Verification items for this drawing (mm, ordinates from the low corner). A direction names the side the tool comes from. Round coordinates to 2 decimals unless told otherwise and drop trailing zeros. Loops run counter-clockwise (first coordinate to the right, second up) from the corner with the lowest first, then second, coordinate; pieces in that order, holes last. Notation, with made-up numbers: (-27.75, 78.5) - (-13.75, 78.5) arc R16 cw to (-13.75, 109.5) - close; hole circle Ø3 at (48, 9). An arc over 180 degrees is marked (long way). Write item = value, one per line.
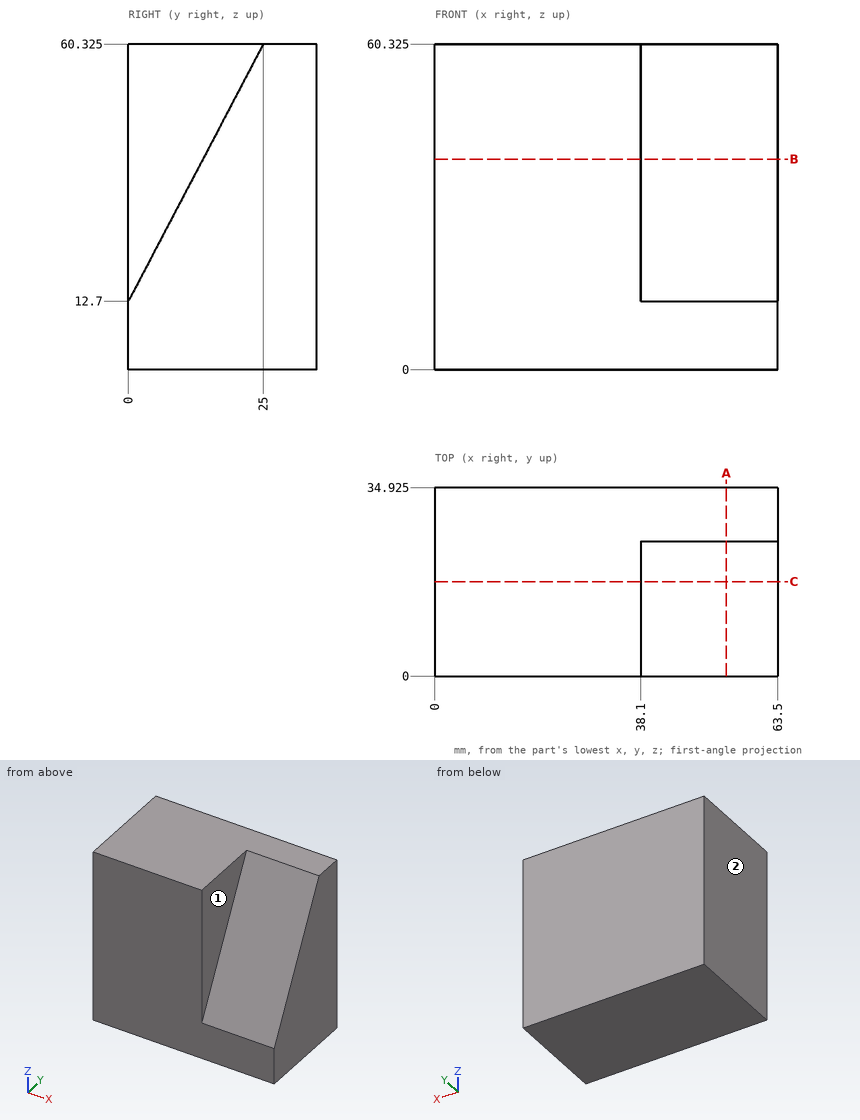
(1) Scan lines: L1, parallel to X at y = 21, z = 54; L2, parallel to Y at x = 41.5, z = 34 (1 decimal); L3, parallel to Y at x = 59, z = 18.5 (1 decimal). Record each from-to range of solid material in increasing order. Write a range as [from, to].
Answers follow:
L1 = [0, 38.1]
L2 = [11.2, 34.9]
L3 = [3, 34.9]
(2) Gauge pin test, flat ends, axial feed: pin 1 (5 mm diameter, centred on y = 17.5, z = 54, fed in from +X); pin 2 (2 mm diameter, centred on x = 47, z = 28.5, fed in from -Y). Record the tip position at first contact, or that the pin passes through.
Answers follow:
pin_1 = 38.1
pin_2 = 7.77
(3) Set-up check for the marked faces 1 and 2: record each of +Z, -Z, +X, -X, +Y, -Y from which the full face is reachable in a straight line by a thin tool's end or side.
Answers follow:
face_1 = +Z, +X, -Y
face_2 = +Z, -Z, -X, +Y, -Y
(4) Section check C-C (y = 17.5). Enter the section's corners in (x, z) (1 decimal).
Answers follow:
outline = (0, 0) - (63.5, 0) - (63.5, 46) - (38.1, 46) - (38.1, 60.3) - (0, 60.3) - close
(5) Section check A-A (x = 54). Enter the section's corners in (y, z) (3 decimals).
Answers follow:
outline = (0, 0) - (34.925, 0) - (34.925, 60.325) - (25, 60.325) - (0, 12.7) - close
(6) Section check B-B (z = 39). Enter the section's corners in (x, y) (3 decimals).
Answers follow:
outline = (0, 0) - (38.1, 0) - (38.1, 13.806) - (63.5, 13.806) - (63.5, 34.925) - (0, 34.925) - close
